Could you check a few things on this drawing? It's one solid part, dimensions in mm from its lowest x, y, z. A direction names the side the tool comes from. Give positions to 0.01 mm unless a question says otherwise; leave off trailing zeros. Loops run counter-clockwise (first coordinate to the right, second up) from the corner with the lowest first, then second, coordinate; pieces in that order, holes last. Notation, with made-up numbers: (-11.5, 26.25) - (6.5, 26.25) arc R31 ccw to (6.5, 53.25) - close; hole circle Ø9 at (30, 50.5). An arc over 180 degrees is marked (long way). Use a Markdown table: item, result.
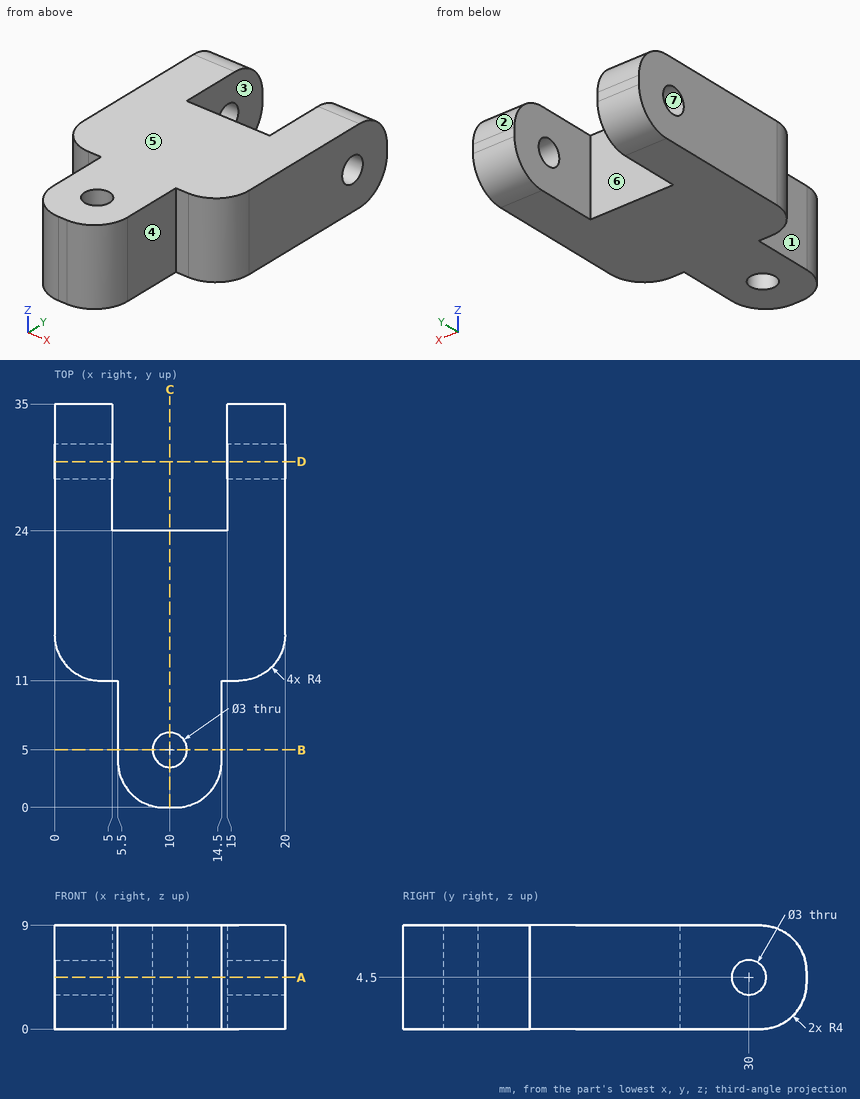
(1) On a 3-axis mill with a long thin cutter (end or side, diameter ignored), from which of +Z, -Z, +X, -X, +Y, -Y can I reach the whole of each face in a straight line? I mean the marked faces 1, 2, 3 and 4. Say none if no direction works.
A:
| item | result |
|---|---|
| face 1 | +Z, -Z, -X, -Y |
| face 2 | +Z, +X, -X, +Y |
| face 3 | +Z, -Z, +Y |
| face 4 | +Z, -Z, +X, -Y |
(2) If I drill on line 1 (Z direction, x = 2.2, y = 30); line 2 (Y direction, x = 10, z = 6); line 3 (X direction, y = 27, z = 5), over which ranges is the centre line in solid material (lowest first)?
A:
| item | result |
|---|---|
| line 1 | 0 to 3, 6 to 9 |
| line 2 | 0 to 3.5, 6.5 to 24 |
| line 3 | 0 to 5, 15 to 20 |
(3) Suppose I cut it at B-B on y = 5. Write out the boundary of the cut face in (x, z), plus the area to 3 significant figures.
A:
| item | result |
|---|---|
| outline | (5.5, 0) - (8.5, 0) - (8.5, 9) - (5.5, 9) - close; (11.5, 0) - (14.5, 0) - (14.5, 9) - (11.5, 9) - close |
| area | 54.0 mm2 |
(4) We'd pull the mould along Y, two halves only. Please class the marked faces 5, 6 and 7: pulls with the +Y half, pulls with the -Y half, needs draft (parallel to the pull), parting line crosses it, or undercut.
A:
| item | result |
|---|---|
| face 5 | needs draft |
| face 6 | pulls with the +Y half |
| face 7 | undercut |
(5) Suppose I cut it at A-A on z = 4.5. Write out the boundary of the cut face in (x, y), plus the area to 3 significant figures.
A:
| item | result |
|---|---|
| outline | (0, 15) arc R4 ccw to (4, 11) - (5.5, 11) - (5.5, 4) arc R4 ccw to (9.5, 0) - (10.5, 0) arc R4 ccw to (14.5, 4) - (14.5, 11) - (16, 11) arc R4 ccw to (20, 15) - (20, 28.5) - (15, 28.5) - (15, 24) - (5, 24) - (5, 28.5) - (0, 28.5) - close; (0, 31.5) - (5, 31.5) - (5, 35) - (0, 35) - close; (15, 31.5) - (20, 31.5) - (20, 35) - (15, 35) - close; hole circle Ø3 at (10, 5) |
| area | 418 mm2 |
(6) Suppose I cut it at D-D on y = 30. Write out the boundary of the cut face in (x, z).
A:
| item | result |
|---|---|
| outline | (0, 0) - (5, 0) - (5, 3) - (0, 3) - close; (0, 6) - (5, 6) - (5, 9) - (0, 9) - close; (15, 0) - (20, 0) - (20, 3) - (15, 3) - close; (15, 6) - (20, 6) - (20, 9) - (15, 9) - close |
(7) Suppose I cut it at C-C on x = 10. Write out the boundary of the cut face in (y, z).
A:
| item | result |
|---|---|
| outline | (0, 0) - (3.5, 0) - (3.5, 9) - (0, 9) - close; (6.5, 0) - (24, 0) - (24, 9) - (6.5, 9) - close |
(8) Will these pins go through, and if not, where does the flat tip stop? pin 1 (0.8 mm diameter, centred on x = 4.5, z = 4, fed in from -Y); pin 2 (1 mm diameter, centred on x = 18, y = 10.5, fed in from -Z); pin 3 (1 mm diameter, centred on y = 11.5, z = 4, fed in from +X); pin 4 (4.5 mm diameter, centred on x = 10.5, z = 3.5, fed in from +Y).
A:
| item | result |
|---|---|
| pin 1 | y = 11 |
| pin 2 | through |
| pin 3 | x = 18.65 |
| pin 4 | y = 24 |
